Check sheet for the modelled part. Datum: model origin and axes. Units: mm. Face numbers are marked on the shaded views. A direction names the side the tool comes from. Round coordinates to 2 decimals unless told otherwise and drop trailing zeros. Loops run counter-clockwise (first coordinate to the right, second up) from the corner with the lowest first, then second, coordinate; pieces in that order, holes last. Notation, with made-up numbers: (54.25, 11) - (98.25, 11) arc R17 ccw to (98.25, 21) - close; hole circle Ø8 at (-7.5, 77.25). An arc over 180 degrees is marked (long way). Return JSON: item names as keys, results as strings.
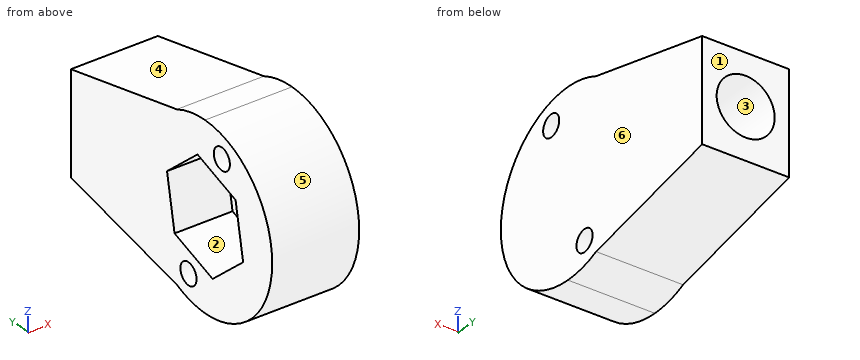
from build123d import *

# Parameters (mm, degrees)
F1_DEPTH = 12
F2_R     = 4
F3_DEPTH = 10
F4_R     = 7.55
F5_DEPTH = 4
F6_R     = 1.5
F7_DEPTH = 25


with BuildPart() as f1:
    # F0 (on Right) → F1 (new body)
    with BuildSketch(Plane.YZ):
        with BuildLine():
            Line((5.246089, 11.34586), (0, 12.5))
            ThreePointArc((0, 12.5), (-12.5, 0), (0, -12.5))
            Line((0, -12.5), (5.246089, -11.34586))
            ThreePointArc((5.246089, -11.34586), (10.531527, -6.733271), (12.5, 0))
            ThreePointArc((12.5, 0), (10.531527, 6.733271), (5.246089, 11.34586))
        make_face()
        Polygon((7.088382, 2.467421), (5.681041, -4.905009), (-1.407342, -7.37243), (-7.088382, -2.467421), (-5.681041, 4.905009), (1.407342, 7.37243), align=None, mode=Mode.SUBTRACT)
        with BuildLine():
            ThreePointArc((5.246089, 11.34586), (2.685772, 12.208056), (0, 12.5))
            Line((0, 12.5), (5.246089, 11.34586))
        make_face()
        with BuildLine():
            Line((5.246089, -11.34586), (0, -12.5))
            ThreePointArc((0, -12.5), (2.685772, -12.208056), (5.246089, -11.34586))
        make_face()
        with BuildLine():
            Line((25, 7), (5.246089, 11.34586))
            ThreePointArc((5.246089, 11.34586), (10.531527, 6.733271), (12.5, 0))
            ThreePointArc((12.5, 0), (10.531527, -6.733271), (5.246089, -11.34586))
            Line((5.246089, -11.34586), (25, -7))
            Line((25, -7), (25, 0))
            Line((25, 0), (25, 7))
        make_face()
    extrude(amount=F1_DEPTH)

    # F2 (on face) → F3 (cut)
    with BuildSketch(Plane(origin=(0, 25, 0), x_dir=(-1, 0, 0), z_dir=(0, 1, 0))):
        with Locations((-6, 0)):
            Circle(F2_R)
    extrude(amount=-F3_DEPTH, mode=Mode.SUBTRACT)

    # F4 (on face) → F5 (join)
    with BuildSketch(Plane.YZ.offset(12)):
        Circle(F4_R)
    extrude(amount=-F5_DEPTH)

    # F6 (on face) → F7 (cut)
    with BuildSketch(Plane(origin=(0, 0, 0), x_dir=(0, -1, 0), z_dir=(-1, 0, 0))):
        with Locations((3.123088, 8.971974)):
            Circle(F6_R)
        with Locations((-3.089254, -8.874777)):
            Circle(F6_R)
    extrude(amount=-F7_DEPTH, mode=Mode.SUBTRACT)


solid = f1.part
Q1. Depth check by flat-ended pin: P1, Ø2, axis at x = 1.5, z = 8.5, coming from the -Y side; P2, Ø4, axis at y = -3.12, z = 8.97, coming from the +X side; P3, Ø2, axis at x = 9, y = 20, coming from the -Z side; P4, Ø3, axis at x = 3.5, y = -4, coming from the +Z side. Enter the tip coordinate at first touch or a pass-through.
Answer key:
{"P1": "stops at y = -10", "P2": "stops at x = 12", "P3": "stops at z = -8.32", "P4": "stops at z = 12.25"}
Q2. Tool access check on the marked faces 1 and 2. Record the directions out of +Z, -Z, +X, -X, +Y, -Y that give a thin tool (end or side, any length) a straight path to the whole face; none if there is none.
Answer key:
{"face 1": "+Z, -Z, +X, -X, +Y", "face 2": "-X"}
Q3. Sectioned sample at A-A (y = 19). Enter the section's corners in (x, z).
Answer key:
{"outline": "(0, -8.32) - (12, -8.32) - (12, 8.32) - (0, 8.32) - close; hole circle Ø8 at (6, 0)"}
Q4. Sectioned sample at B-B (x = 6.5). Enter the section's corners in (y, z) (3 decimals).
Answer key:
{"outline": "(0, -12.5) arc R12.5 ccw to (5.246, -11.346) - (25, -7) - (25, -3.969) - (15, -3.969) - (15, 3.969) - (25, 3.969) - (25, 7) - (5.246, 11.346) arc R12.5 ccw to (0, 12.5) arc R12.5 ccw to start; hole (-7.088, -2.467) - (-1.407, -7.372) - (5.681, -4.905) - (7.088, 2.467) - (1.407, 7.372) - (-5.681, 4.905) - close; hole circle Ø3 at (-3.123, 8.972); hole circle Ø3 at (3.089, -8.875)"}
Q5. Sectioned sample at D-D (x = 11). Enter the section's corners in (y, z), plus the area to 3 significant figures.
Answer key:
{"outline": "(0, -12.5) arc R12.5 ccw to (5.25, -11.35) - (25, -7) - (25, 7) - (5.25, 11.35) arc R12.5 ccw to (0, 12.5) arc R12.5 ccw to start; hole circle Ø3 at (-3.12, 8.97); hole circle Ø3 at (3.09, -8.87)", "area": "721 mm²"}
Q6. Scan lines: probe 1 along Z at (x, y) = (3.25, -3.5); probe 2 along Z at (x, y) = (8.25, 17); probe 3 along Z at (x, y) = (6, 21.5). Record each from-to range of solid material in increasing order. Write a range as [from, to].
Answer key:
{"probe 1": "z = [-12, -5.57], [5.66, 7.52], [10.42, 12]", "probe 2": "z = [-8.76, -3.31], [3.31, 8.76]", "probe 3": "z = [-7.77, -4], [4, 7.77]"}
Q7. Sectioned sample at C-C (z = 0). Enter the section's corners in (x, y), plus the area to 3 significant figures.
Answer key:
{"outline": "(0, -12.5) - (12, -12.5) - (12, 25) - (10, 25) - (10, 15) - (2, 15) - (2, 25) - (0, 25) - (0, 6.62) - (8, 6.62) - (8, -6.62) - (0, -6.62) - close", "area": "264 mm²"}
Q8. Draft check along Z on the marked faces 3, 4, 5 and 6. Enter one of: released by +Z, released by -Z, zero draft, split by the parting line, or undercut.
Answer key:
{"face 3": "undercut", "face 4": "released by +Z", "face 5": "split by the parting line", "face 6": "zero draft"}
